The listing builds one solid part. Answer for the finished solid, in the listing's coordinates (mm). Give positions to 0.01 mm unless a question says otherwise; leave off trailing zeros. Use a Markdown table: item, result. Add a question column.
1) Flat-ended cylindrical pins translate along their axes: pin 1 (8 mm diameter, centred on x = 118.5, y = 333, fed in from -Z); pin 2 (6 mm diameter, centred on x = 158.5, y = 201.5, fed in from +Z); pin 3 (5 mm diameter, centred on x = 194, y = 135.5, fed in from +Z). Find the tip coordinate at first contact, or state that the pin passes through.
2) Straight lines are drawn through the part: line 1 (X direction, y = 347.5, z = -5.5); line 2 (Y direction, x = 213, z = 0.25); line 3 (Z direction, x = 134.5, y = 273.5). For each, find the intervals that lie inside material, in ascending order.
3) Find section A-A, the plane y = 312.5. State how many separate pieces and enclosed holes the cut face has, plus the area to 3 significant figures.
from build123d import *

# Parameters (mm, degrees)
F1_W     = 15
F1_H     = 15
F3_R     = 3
F4_DEPTH = 450


with BuildPart() as f2:
    # F2: sweep along a path in F0
    with BuildLine(Plane.XY) as f2_path:
        Line((0, 0), (560, 0))
        Line((560, 0), (560, 465))
        Line((560, 465), (0, 465))
        Line((0, 465), (0, 0))
    # F1 (on Right) → F2 (sweep)
    with BuildSketch(Plane.YZ):
        Rectangle(F1_W, F1_H)
    sweep(path=f2_path.line, transition=Transition.RIGHT)

    # F3 (on face) → F4 (join)
    with BuildSketch(Plane.XZ.offset(-457.5)):
        with Locations((25.66667, 0)):
            Circle(F3_R)
        with Locations((43.83334, 0)):
            Circle(F3_R)
        with Locations((62.00001, 0)):
            Circle(F3_R)
        with Locations((80.16668, 0)):
            Circle(F3_R)
        with Locations((98.33335, 0)):
            Circle(F3_R)
        with Locations((116.50002, 0)):
            Circle(F3_R)
        with Locations((134.66669, 0)):
            Circle(F3_R)
        with Locations((152.83336, 0)):
            Circle(F3_R)
        with Locations((171.00003, 0)):
            Circle(F3_R)
        with Locations((189.1667, 0)):
            Circle(F3_R)
        with Locations((207.33337, 0)):
            Circle(F3_R)
        with Locations((225.50004, 0)):
            Circle(F3_R)
        with Locations((243.66671, 0)):
            Circle(F3_R)
        with Locations((261.83338, 0)):
            Circle(F3_R)
        with Locations((280.00005, 0)):
            Circle(F3_R)
        with Locations((298.16672, 0)):
            Circle(F3_R)
        with Locations((316.33339, 0)):
            Circle(F3_R)
        with Locations((334.50006, 0)):
            Circle(F3_R)
        with Locations((352.66673, 0)):
            Circle(F3_R)
        with Locations((370.8334, 0)):
            Circle(F3_R)
        with Locations((389.00007, 0)):
            Circle(F3_R)
        with Locations((407.16674, 0)):
            Circle(F3_R)
        with Locations((425.33341, 0)):
            Circle(F3_R)
        with Locations((443.50008, 0)):
            Circle(F3_R)
        with Locations((461.66675, 0)):
            Circle(F3_R)
        with Locations((479.83342, 0)):
            Circle(F3_R)
        with Locations((498.00009, 0)):
            Circle(F3_R)
        with Locations((516.16676, 0)):
            Circle(F3_R)
        with Locations((534.33343, 0)):
            Circle(F3_R)
    extrude(amount=F4_DEPTH)


solid = f2.part
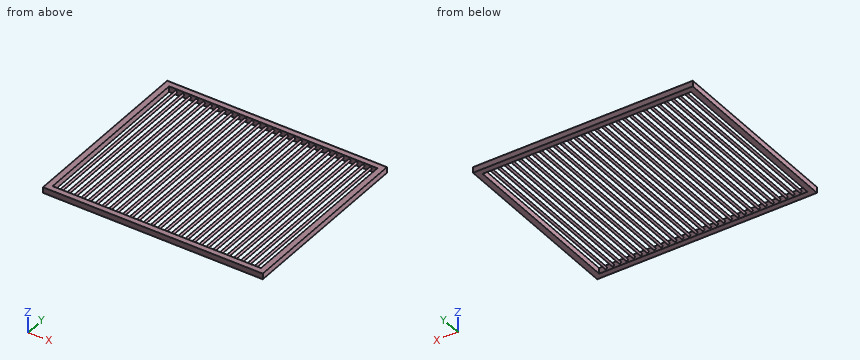
The answers:
| question | item | result |
|---|---|---|
| 1 | pin 1 | z = -3 |
| 1 | pin 2 | z = 1.37 |
| 1 | pin 3 | z = 1.89 |
| 2 | line 1 | -7.5 to 7.5, 552.5 to 567.5 |
| 2 | line 2 | -7.5 to 7.5, 457.5 to 472.5 |
| 2 | line 3 | -3 to 3 |
| 3 | separate pieces | 31 |
| 3 | enclosed holes | 0 |
| 3 | area | 1,270 mm2 |
